Check sheet for the drawn part. Datum: minimum x, y, z corner. Units: mm. A direction names the side the tool comes from. Give positions to 0.01 mm unless a question says otherwise; leave off trailing zeros. Write each loop counter-clockwise with the first axis right and the second up, starting at its lowest first coordinate (ties: lowest second). Pieces come first, ordered by that corner, then holes. Notation, with made-up numbers: (54.25, 51.5) -> (91.25, 51.5) arc R28 ccw to (91.25, 84.5) -> close; hole circle Ø10 at (39.25, 23). An arc over 180 degrees is marked (long way). Write item = value, one per line. Start each with the question number.
1. Thickness scan on line 1 along X through (y, z) = (41, 58) (3 decimals); line 2 along Z through (x, y) = (36, 42). Record the ranges inside material, lowest first.
2. Cross-section at A-A, the plane x = 49. Record the cut outline in (y, z) (3 decimals), plus the area to 3 significant figures.
3. Cross-section at C-C, the plane y = 10. Record the cut outline in (x, z) (3 decimals).
4. Depth check by flat-ended pin: P1, Ø6, axis at x = 52.5, y = 40.5, coming from the +Z side; P2, Ø6, axis at x = 12.5, z = 30, coming from the -Y side (3 decimals). Enter the tip coordinate at first touch or a pass-through.
5. Mould release check, pull along Y, two halves, no side actions. Record for the marked faces 3, 4 and 5: pulls with the +Y half, pulls with the -Y half, needs draft (parallel to the pull), parting line crosses it, or undercut.
6. Cross-section at B-B, the plane z = 39.5. Record the cut outline in (x, y) (3 decimals), plus the area to 3 significant figures.
7. Set-up check for the marked faces 1 and 2: record each of +Z, -Z, +X, -X, +Y, -Y from which the full face is reachable in a straight line by a thin tool's end or side.
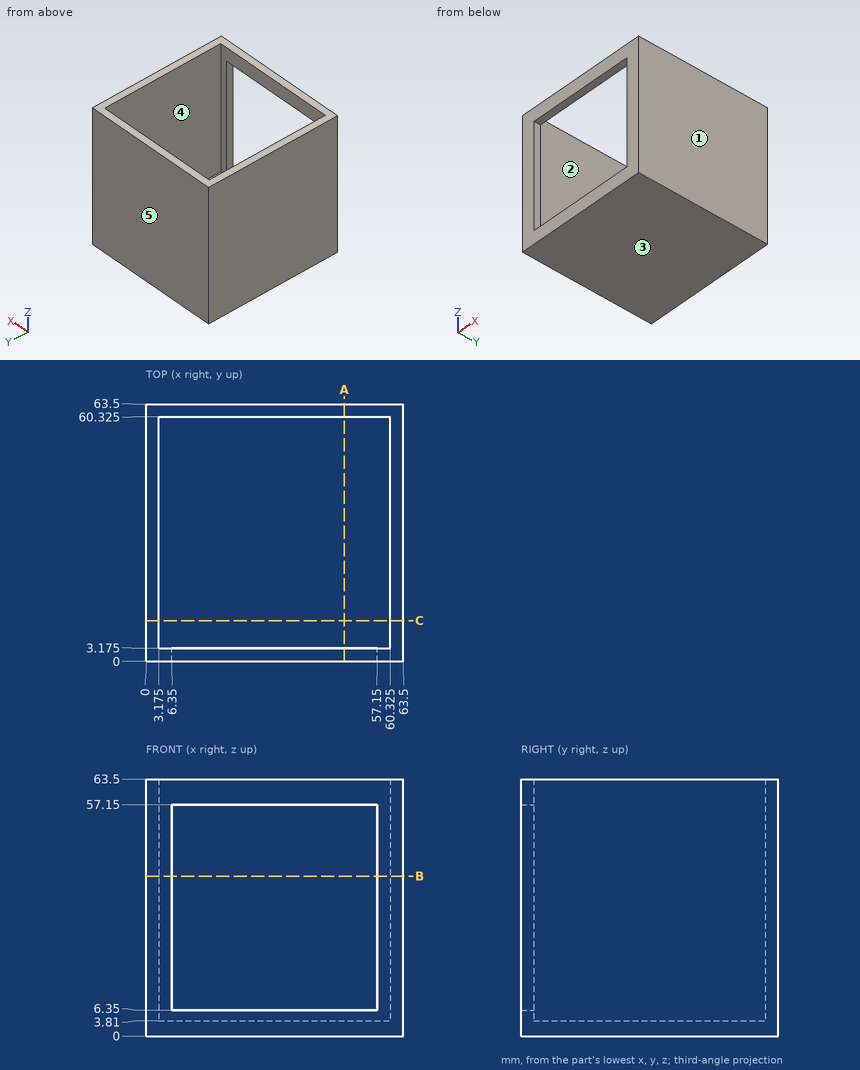
Answers:
q1.line_1 = 0 to 3.175, 60.325 to 63.5
q1.line_2 = 0 to 3.81
q2.outline = (0, 0) -> (63.5, 0) -> (63.5, 63.5) -> (60.325, 63.5) -> (60.325, 3.81) -> (3.175, 3.81) -> (3.175, 6.35) -> (0, 6.35) -> close; (0, 57.15) -> (3.175, 57.15) -> (3.175, 63.5) -> (0, 63.5) -> close
q2.area = 460 mm^2
q3.outline = (0, 0) -> (63.5, 0) -> (63.5, 63.5) -> (60.325, 63.5) -> (60.325, 3.81) -> (3.175, 3.81) -> (3.175, 63.5) -> (0, 63.5) -> close
q4.P1 = 3.81
q4.P2 = 60.325
q5.face_3 = needs draft
q5.face_4 = undercut
q5.face_5 = pulls with the +Y half
q6.outline = (0, 0) -> (6.35, 0) -> (6.35, 3.175) -> (3.175, 3.175) -> (3.175, 60.325) -> (60.325, 60.325) -> (60.325, 3.175) -> (57.15, 3.175) -> (57.15, 0) -> (63.5, 0) -> (63.5, 63.5) -> (0, 63.5) -> close
q6.area = 605 mm^2
q7.face_1 = +Z, -Z, +X, +Y, -Y
q7.face_2 = +Z
